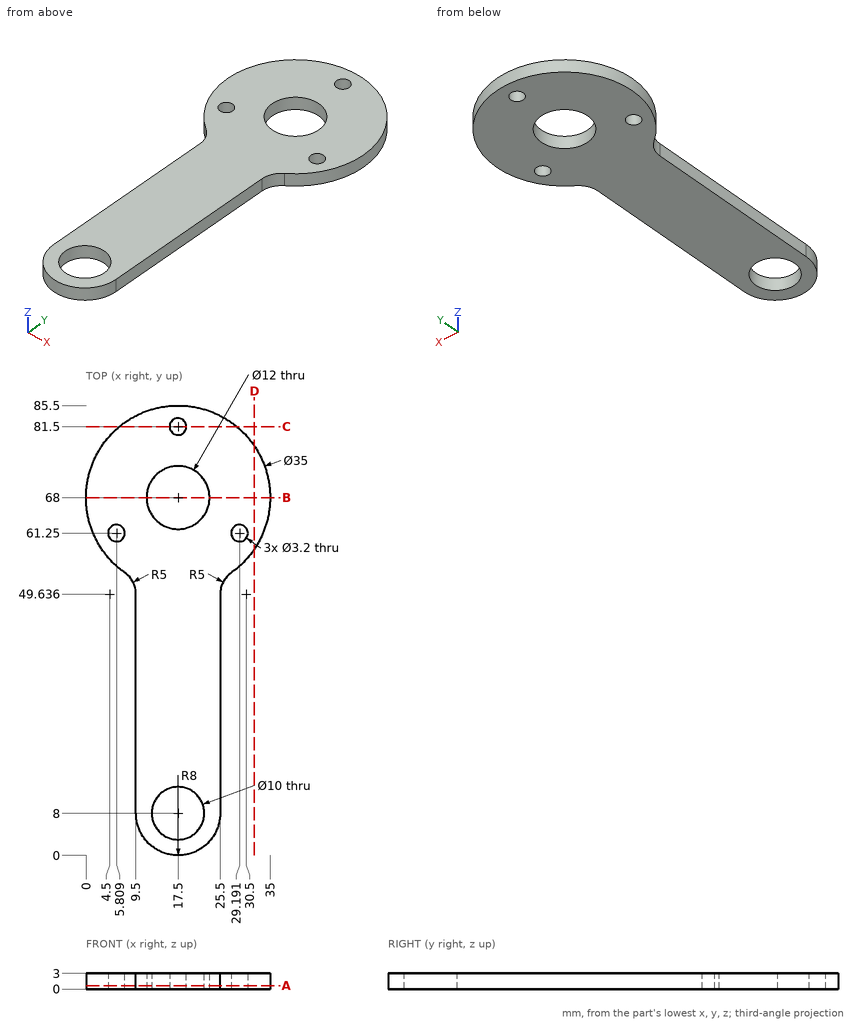
Part print with two shaded views. Sizes in mm from the minimum x, y, z corner. Round coordinates to 2 decimals unless told otherwise and drop trailing zeros. Order: outer loops, then holes, each group sorted by start corner. A loop starts at its lowest first (then second) coordinate and runs counter-clockwise, first axis right, second up. Notation, with made-up numbers: (68, 48) - (76, 48) arc R26 ccw to (76, 62) - close; hole circle Ø3 at (-4.5, 54). An arc over 180 degrees is marked (long way). Answer as CSV lines item,"result". Start each with the question number.
1. Saw through at A-A, the plane z = 0.65. Count the separate pieces of the cut face and the enclosed holes in it, and give its area (3 significant figures).
2. Saw through at B-B, the plane y = 68. Write the cut outline in (x, z).
3. Saw through at D-D, the plane x = 32. Write the cut outline in (y, z), and give its area (3 significant figures).
4. Saw through at C-C, the plane y = 81.5. Write the cut outline in (x, z) (1 decimal).
5. Pin check, flat tips, straight feed: pin 1 (1.5 mm diameter, centred on y = 20.5, z = 1.5, fed in from -X); pin 2 (1.5 mm diameter, centred on y = 73, z = 2.5, fed in from -X); pin 3 (0.9 mm diameter, centred on y = 31, z = 1.5, fed in from +X). Stop position of each tip, or through.
6. Drill centre lines: L1, parallel to Y at x = 17.5, z = 1.25; L2, parallel to Y at x = 15, z = 2.5 (1 decimal); L3, parallel to X at y = 61.25, z = 1.2 (1 decimal). Where is each one in solid material? Low to high. Write a range as [from, to].
Model answer:
1,separate pieces,"1"
1,enclosed holes,"5"
1,area,"1,540 mm²"
2,outline,"(0, 0) - (11.5, 0) - (11.5, 3) - (0, 3) - close; (23.5, 0) - (35, 0) - (35, 3) - (23.5, 3) - close"
3,outline,"(58.2, 0) - (77.8, 0) - (77.8, 3) - (58.2, 3) - close"
3,area,"58.8 mm²"
4,outline,"(6.4, 0) - (15.9, 0) - (15.9, 3) - (6.4, 3) - close; (19.1, 0) - (28.6, 0) - (28.6, 3) - (19.1, 3) - close"
5,pin 1,"stops at x = 9.5"
5,pin 2,"stops at x = 0.52"
5,pin 3,"stops at x = 25.5"
6,L1,"y = [0, 3], [13, 62], [74, 79.9], [83.1, 85.5]"
6,L2,"y = [0.4, 3.7], [12.3, 62.5], [73.5, 85.3]"
6,L3,"x = [1.4, 4.2], [7.4, 27.6], [30.8, 33.6]"
